Could you check a few things on this model? Use its own coordinates, in mm. Face numbers are marked on the shaded views. A direction names the side the tool comes from. Round coordinates to 2 decimals unless told otherwise and drop trailing zeros. Loops run counter-clockwise (first coordinate to the right, second up) from the corner with the lowest first, then second, coordinate; pieces in that order, holes last. Notation, with made-up numbers: M 89.25,53.5 L 141.25,53.5 A18 cw 141.25,60.5 Z; hole C 41,31.5 d2. An arc over 180 degrees is marked long. Answer in a Markdown table with one row per item.
```python
from build123d import *

# Parameters (mm, degrees)
SKETCH2_W               = 1.9
SKETCH2_H               = 1.4
CUT_EXTRUDE1_DEPTH      = 7
CUT_EXTRUDE1_DEPTH_BACK = 7


with BuildPart() as part:
    # Sketch1 → Revolve1 (revolve)
    with BuildSketch(Plane.XY):
        with BuildLine():
            Line((0, 0), (2, 0))
            Line((2, 0), (2, 1))
            Line((2, 1), (3, 1))
            Line((3, 1), (3, 8))
            Line((3, 8), (6, 8))
            Line((6, 8), (6, 9.1))
            ThreePointArc((6, 9.1), (5.267766953, 10.867766953), (3.5, 11.6))
            Line((3.5, 11.6), (0, 11.6))
            Line((0, 11.6), (0, 0))
        make_face()
    revolve(axis=Axis((0, 0, 0), (0, 1, 0)))

    # Sketch2 → Cut-Extrude1 (cut, two sides)
    with BuildSketch(Plane.XY) as cut_extrude1_sk:
        with Locations((0, 10.9)):
            Rectangle(SKETCH2_W, SKETCH2_H)
    extrude(amount=CUT_EXTRUDE1_DEPTH, mode=Mode.SUBTRACT)
    extrude(cut_extrude1_sk.sketch, amount=-CUT_EXTRUDE1_DEPTH_BACK, mode=Mode.SUBTRACT)


solid = part.part
```
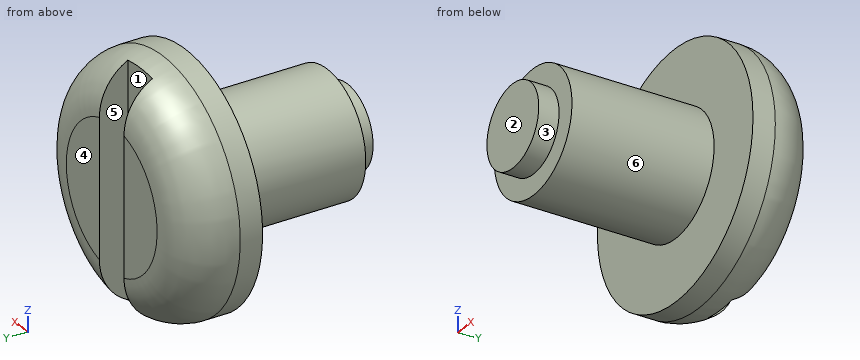
1) If we mould it in two halves opening along X, with no side actions, what happens to the marked faces 1, 2 and 3? For each: released by +X, released by -X, zero draft, split by the parting line, or undercut.
Computed:
| item | result |
|---|---|
| face 1 | undercut |
| face 2 | zero draft |
| face 3 | split by the parting line |
2) I want a section at C-C, the plane y = 8.75. Please give me the cut outline in (x, z).
Computed:
| item | result |
|---|---|
| outline | C 0,0 d12 |
3) I want a section at D-D, the plane y = 7. Please give me the cut outline in (x, z), plus the area to 3 significant figures.
Computed:
| item | result |
|---|---|
| outline | C 0,0 d6 |
| area | 28.3 mm² |
4) Which directions (+Z, -Z, +X, -X, +Y, -Y) give clear straight access to the entire face, cutting with the end or side of a thin tool? Please do the marked faces 4, 5 and 6.
Computed:
| item | result |
|---|---|
| face 4 | +Z, -Z, +X, -X, +Y |
| face 5 | +Z, -Z, +Y |
| face 6 | -Y |
5) I want a section at B-B, the plane x = 0. Please give me the cut outline in (y, z) (3 decimals), plus the area to 3 significant figures.
Computed:
| item | result |
|---|---|
| outline | M 0,-2 L 1,-2 L 1,-3 L 8,-3 L 8,-6 L 9.1,-6 A2.5 ccw 10.2,-5.745 L 10.2,5.745 A2.5 ccw 9.1,6 L 8,6 L 8,3 L 1,3 L 1,2 L 0,2 Z |
| area | 72.2 mm² |
6) Will these pins go through, and if not, where does the flat tip stop? P1, Ø2, axis at y = 8, z = -2, coming from the -X side; P2, Ø1.1, axis at y = 10.5, z = 0, coming from the +X side; P3, Ø1.5, axis at x = -1.5, y = 8.5, coming from the +Z side.
Computed:
| item | result |
|---|---|
| P1 | stops at x = -5.92 |
| P2 | stops at x = 5.85 |
| P3 | stops at z = 5.95 |
7) I need wall thicknesses on line 1 (Y direction, x = -0.75, z = 4.75); line 2 (X direction, y = 8.25, z = -1); line 3 (Z direction, x = 4, y = 10.25). Which ranges of each line are inside material? Lowest first, please.
Computed:
| item | result |
|---|---|
| line 1 | y = 8 to 10.2 |
| line 2 | x = -5.92 to 5.92 |
| line 3 | z = -4.09 to 4.09 |
8) I want a section at A-A, the plane z = 0. Please give me the cut outline in (x, y), plus the area to 3 significant figures.
Computed:
| item | result |
|---|---|
| outline | M -6,8 L -3,8 L -3,1 L -2,1 L -2,0 L 2,0 L 2,1 L 3,1 L 3,8 L 6,8 L 6,9.1 A2.5 ccw 3.5,11.6 L 0.95,11.6 L 0.95,10.2 L -0.95,10.2 L -0.95,11.6 L -3.5,11.6 A2.5 ccw -6,9.1 Z |
| area | 83.9 mm² |
